Read the model definition and answer for the solid it produces. Units are mm, in the model's axes. Face numbers are marked on the shaded views. A direction names the side the tool comes from. Give positions to 0.01 mm unless a question says otherwise; leave off trailing zeros. Loops run counter-clockwise (first coordinate to the right, second up) from the corner with the lowest first, then second, coordinate; pieces in that order, holes last. Notation, with made-up numbers: M 38.25,16.5 L 57.25,16.5 A18 cw 57.25,31.5 Z; hole C -12,-32.5 d2. An arc over 180 degrees is marked long. Return JSON: item names as keys, results as strings. Group by question number.
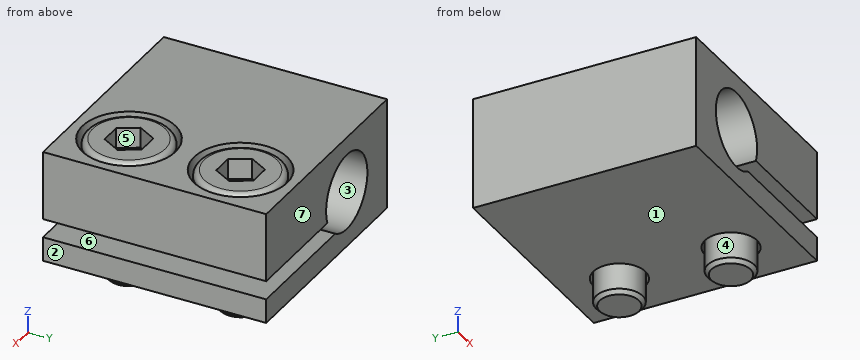
Autodesk Inventor part; units mm, degrees
ref_plane "as_nhs_01_XY" through (9, 3, 0) normal (0, 0, 1) x (1, 0, 0)
ref_plane "as_nhs_01_YZ" through (9, 3, 0) normal (1, 0, 0) x (0, 1, 0)
ref_plane "as_nhs_01_ZX" through (9, 3, 0) normal (0, 1, 0) x (0, 0, 1)
sketch "Sketch_1" plane through (0, 0, 0) normal (0, 1, 0) x (-1, 0, 0)
  line L0 (0, 6) -> (-12, 6)
  line L1 (-12, 6) -> (-12, 2.3)
  line L2 (-12, 2.3) -> (-5.9268, 2.3)
  arc A0 (-5.1456, 1.3) -> (-5.9268, 2.3) centre (-4, 3) ccw
  line L3 (-5.1456, 1.3) -> (-12, 1.3)
  line L4 (-12, 1.3) -> (-12, 0)
  line L5 (-12, 0) -> (0, 0)
  line L6 (0, 0) -> (0, 6)
extrude "Extrusion1" add sketch "Sketch_1" along normal blind 12
sketch "Sketch2" plane through (12, 0, 0) normal (0, 0, -1) x (-1, 0, 0)
  point P0 (3, 3)
hole "Hole1" at (9, 3, 0) direction (0, 0, 1) diameter 2.8 depth 6
pattern_linear "Rectangular Pattern1" count 2 spacing 6 along (0, 1, 0) of "Hole1"
sketch "Sketch_4" plane through (9, 0, 0) normal (1, 0, 0) x (0, 0, -1)
  line L0 (-3.5, 3) -> (-6, 3)
  line L1 (-6, 3) -> (-6, 5.5)
  line L2 (-6, 5.5) -> (-3.5, 5.5)
  line L3 (-3.5, 5.5) -> (-3.5, 3)
  line L4 (-3.5, 3) -> (-6, 3)
revolve "Revolution1" cut sketch "Sketch_4" angle 360 about axis through (9, 3, 3.5) along (0, 0, -1)
pattern_linear "Rectangular Pattern2" count 2 spacing 6 along (0, 1, 0) of "Revolution1"
sketch "Sketch_12" plane through (9, 0, 0) normal (1, 0, 0) x (0, 0, -1)
  line L0 (1.5, 3) -> (-6, 3)
  line L1 (-6, 3) -> (-6, 4.95)
  arc A0 (-5.7, 5.25) -> (-6, 4.95) centre (-5.7, 4.95) ccw
  line L2 (-5.7, 5.25) -> (-3.5, 5.25)
  line L3 (-3.5, 5.25) -> (-3.5, 4.25)
  line L4 (-3.5, 4.25) -> (1.3, 4.25)
  line L5 (1.3, 4.25) -> (1.5, 4.05)
  line L6 (1.5, 4.05) -> (1.5, 3)
  line L7 (1.5, 3) -> (-6, 3)
revolve "Revolution2" add sketch "Sketch_12" angle 360 about axis through (9, 3, -1.5) along (0, 0, -1)
thread "Thread1"
pattern_linear "Rectangular Pattern3" count 2 spacing 6 along (0, 1, 0) of "Revolution2"
sketch "Sketch_14" plane through (9, 3, 6) normal (0, 0, 1) x (0, 1, 0)
  line L0 (-1, -0.5774) -> (0, -1.1547)
  line L1 (0, -1.1547) -> (1, -0.5774)
  line L2 (1, -0.5774) -> (1, 0.5774)
  line L3 (1, 0.5774) -> (0, 1.1547)
  line L4 (0, 1.1547) -> (-1, 0.5774)
  line L5 (-1, 0.5774) -> (-1, -0.5774)
extrude "Extrusion2" cut sketch "Sketch_14" against normal blind 1.1
pattern_linear "Rectangular Pattern4" count 2 spacing 6 along (0, 1, 0) of "Extrusion2"
ref_plane "as_nhs_01_XY" through (9, 3, 0) normal (0, 0, 1) x (1, 0, 0)
ref_plane "as_nhs_01_YZ" through (9, 3, 0) normal (1, 0, 0) x (0, 1, 0)
ref_plane "as_nhs_01_ZX" through (9, 3, 0) normal (0, 1, 0) x (0, 0, 1)
ref_plane "as_nhs_02_XY" through (9, 9, 0) normal (0, 0, 1) x (1, 0, 0)
ref_plane "as_nhs_02_YZ" through (9, 9, 0) normal (1, 0, 0) x (0, 1, 0)
ref_plane "as_nhs_02_ZX" through (9, 9, 0) normal (0, 1, 0) x (0, 0, 1)
ref_plane "s01_XY" through (9, 3, 3.5) normal (0, 0, 1) x (1, 0, 0)
ref_plane "s01_YZ" through (9, 3, 3.5) normal (1, 0, 0) x (0, 1, 0)
ref_plane "s01_ZX" through (9, 3, 3.5) normal (0, 1, 0) x (0, 0, 1)
ref_plane "s02_XY" through (9, 9, 3.5) normal (0, 0, 1) x (1, 0, 0)
ref_plane "s02_YZ" through (9, 9, 3.5) normal (1, 0, 0) x (0, 1, 0)
ref_plane "s02_ZX" through (9, 9, 3.5) normal (0, 1, 0) x (0, 0, 1)
properties part number "SCHUNK-9700901 Halter fuer NHS Du 4"
1. Find section A-A (z = 5.25). Write down the section's boundary in (x, y).
2. The mould has two halves that part along Z. Classify the marked faces 1, 2 and 3: +Z half, -Z half, draft (parallel to the pull), parting line (faces both ways), or undercut.
3. For the marked faces 4, 5, 6 and 7, determine the directions among +Z, -Z, +X, -X, +Y, -Y from which every point of the face is accessible in a straight line to the end or side of a thin tool.
4. Find section C-C (x = 9). State how many separate pieces and enclosed holes the cut face has, and give its area (3 significant figures).
5. Find section B-B (z = 0.5). Write down the section's boundary in (x, y).
6. Find section D-D (z = -0.25). Write down the section's boundary in (x, y), and give its area (3 significant figures).
7. Straight lines are drawn through the part: line 1 along Z through (x, y) = (6.5, 6); line 2 along X through (y, z) = (10, 0.25); line 3 along X through (y, z) = (9.5, 3.25). For each, find the intervals that lie inside material, in ascending order.
8. A flat-ended cylindrical pin translates along its axis: P1, Ø1.6, axis at x = 9, y = 3, coming from the +Z side. Find the tip coordinate at first contact, or state that the pin passes through.
Result:
{
 "1": {"outline": "M 0,0 L 12,0 L 12,12 L 0,12 Z; C 9,3 d4.5; C 9,9 d4.5; hole C 9,3 d5; hole C 9,9 d5; hole M 7.85,3 L 8.42,2 L 9.58,2 L 10.15,3 L 9.58,4 L 8.42,4 Z; hole M 7.85,9 L 8.42,8 L 9.58,8 L 10.15,9 L 9.58,10 L 8.42,10 Z"},
 "2": {"face 1": "-Z half", "face 2": "draft", "face 3": "undercut"},
 "3": {"face 4": "-Z", "face 5": "+Z", "face 6": "none", "face 7": "+Z, -Z, +X, -X, +Y"},
 "4": {"separate pieces": "4", "enclosed holes": "0", "area": "63.9 mm2"},
 "5": {"outline": "M 0,0 L 12,0 L 12,12 L 0,12 Z; C 9,3 d2.5; C 9,9 d2.5; hole C 9,3 d2.8; hole C 9,9 d2.8"},
 "6": {"outline": "C 9,3 d2.5; C 9,9 d2.5", "area": "9.82 mm2"},
 "7": {"line 1": "z = 0 to 1.3, 2.3 to 6", "line 2": "x = 0 to 8.02, 8.25 to 9.75, 9.98 to 12", "line 3": "x = 0 to 1.97, 6.03 to 7.69, 7.85 to 10.15, 10.31 to 12"},
 "8": {"P1": "stops at z = 4.9"}
}
